```python
from build123d import *

# Parameters (mm, degrees)
BOSS_EXTRUDE1_DEPTH      = 2
BOSS_EXTRUDE1_DEPTH_BACK = 3
SKETCH1_W                = 120
SKETCH1_H                = 120
SKETCH3_W                = 27.75
SKETCH3_H                = 16.75
BOSS_EXTRUDE4_DEPTH      = 18
SKETCH4_W                = 23.75
SKETCH4_H                = 12.75
CUT_EXTRUDE1_DEPTH       = 18
SKETCH5_R                = 3
BOSS_EXTRUDE5_DEPTH      = 7
SKETCH6_W                = 10
SKETCH6_H                = 5
CUT_EXTRUDE2_DEPTH       = 2
SKETCH7_W                = 10
SKETCH7_H                = 5
CUT_EXTRUDE3_DEPTH       = 2
BOSS_EXTRUDE6_REACH      = 112.411
BOSS_EXTRUDE7_REACH      = 121.478
SKETCH12_W               = 120
SKETCH12_H               = 5
CUT_EXTRUDE4_DEPTH       = 3
SKETCH13_W               = 120
SKETCH13_H               = 5
CUT_EXTRUDE5_DEPTH       = 3
SKETCH14_W               = 114
SKETCH14_H               = 5
CUT_EXTRUDE6_DEPTH       = 3
SKETCH15_W               = 114
SKETCH15_H               = 5
CUT_EXTRUDE7_DEPTH       = 3
BOSS_EXTRUDE8_DEPTH      = 2


with BuildPart() as part:
    # Sketch1 → Boss-Extrude1 (new, two sides: drawn at the far end of the back side and taken through both)
    with BuildSketch(Plane(origin=(0, 0, 0), x_dir=(1, 0, 0), z_dir=(0, 1, 0)).offset(-BOSS_EXTRUDE1_DEPTH_BACK)):
        Rectangle(SKETCH1_W, SKETCH1_H)
    extrude(amount=BOSS_EXTRUDE1_DEPTH + BOSS_EXTRUDE1_DEPTH_BACK)

    # Sketch3 → Boss-Extrude4 (add)
    with BuildSketch(Plane(origin=(0, 0, 0), x_dir=(1, 0, 0), z_dir=(0, 1, 0))):
        with Locations((-43.125, -48.625)):
            Rectangle(SKETCH3_W, SKETCH3_H)
        with Locations((43.125, -48.625)):
            Rectangle(SKETCH3_W, SKETCH3_H)
        with Locations((43.125, 48.625)):
            Rectangle(SKETCH3_W, SKETCH3_H)
        with Locations((-43.125, 48.625)):
            Rectangle(SKETCH3_W, SKETCH3_H)
    extrude(amount=-BOSS_EXTRUDE4_DEPTH)

    # Sketch4 → Cut-Extrude1 (cut)
    with BuildSketch(Plane(origin=(0, 2, 0), x_dir=(1, 0, 0), z_dir=(0, 1, 0))):
        with Locations((-43.125, -48.625)):
            Rectangle(SKETCH4_W, SKETCH4_H)
        with Locations((43.125, -48.625)):
            Rectangle(SKETCH4_W, SKETCH4_H)
        with Locations((43.125, 48.625)):
            Rectangle(SKETCH4_W, SKETCH4_H)
        with Locations((-43.125, 48.625)):
            Rectangle(SKETCH4_W, SKETCH4_H)
    extrude(amount=-CUT_EXTRUDE1_DEPTH, mode=Mode.SUBTRACT)

    # Sketch5 → Boss-Extrude5 (add)
    with BuildSketch(Plane(origin=(0, -18, 0), x_dir=(-1, 0, 0), z_dir=(0, -1, 0))):
        with Locations(Location((48.5, -48.625, 0), (0, 0, 90))):
            Circle(SKETCH5_R)
        with Locations(Location((-48.5, -48.625, 0), (0, 0, 270))):
            Circle(SKETCH5_R)
        with Locations(Location((48.5, 48.625, 0), (0, 0, 270))):
            Circle(SKETCH5_R)
        with Locations(Location((-48.5, 48.625, 0), (0, 0, 270))):
            Circle(SKETCH5_R)
    extrude(amount=BOSS_EXTRUDE5_DEPTH)

    # Sketch6 → Cut-Extrude2 (cut)
    with BuildSketch(Plane(origin=(57, 0, 0), x_dir=(0, 0, -1), z_dir=(1, 0, 0))):
        with Locations((-48.625, -13.5)):
            Rectangle(SKETCH6_W, SKETCH6_H)
        with Locations((48.625, -13.5)):
            Rectangle(SKETCH6_W, SKETCH6_H)
    extrude(amount=-CUT_EXTRUDE2_DEPTH, mode=Mode.SUBTRACT)

    # Sketch7 → Cut-Extrude3 (cut)
    with BuildSketch(Plane.ZY.offset(57)):
        with Locations((48.625, -13.5)):
            Rectangle(SKETCH7_W, SKETCH7_H)
        with Locations((-48.625, -13.5)):
            Rectangle(SKETCH7_W, SKETCH7_H)
    extrude(amount=-CUT_EXTRUDE3_DEPTH, mode=Mode.SUBTRACT)

    # Sketch9 → Boss-Extrude6 (add, up to next)
    with BuildSketch(Plane(origin=(-29.25, 0, 0), x_dir=(0, 0, -1), z_dir=(1, 0, 0)), mode=Mode.PRIVATE) as boss_extrude6_sk1:
        Polygon((57, -3), (55, -3), (56.5, -18), (57, -18), align=None)
    boss_extrude6_tool1 = extrude(boss_extrude6_sk1.sketch, amount=BOSS_EXTRUDE6_REACH, mode=Mode.PRIVATE) - part.part
    # Sketch9 → Boss-Extrude6 (add, up to next)
    with BuildSketch(Plane(origin=(-29.25, 0, 0), x_dir=(0, 0, -1), z_dir=(1, 0, 0)), mode=Mode.PRIVATE) as boss_extrude6_sk2:
        Polygon((-56.5, -18), (-55, -3), (-57, -3), (-57, -18), align=None)
    boss_extrude6_tool2 = extrude(boss_extrude6_sk2.sketch, amount=BOSS_EXTRUDE6_REACH, mode=Mode.PRIVATE) - part.part
    add(boss_extrude6_tool1.solids().sort_by_distance((-29.25, -9, -56.3))[0])
    add(boss_extrude6_tool2.solids().sort_by_distance((-29.25, -9, 56.3))[0])

    # Sketch10 → Boss-Extrude7 (add, up to next)
    with BuildSketch(Plane.XY.offset(-40.25), mode=Mode.PRIVATE) as boss_extrude7_sk1:
        Polygon((-57, -3), (-54, -3), (-56.5, -18), (-57, -18), align=None)
    boss_extrude7_tool1 = extrude(boss_extrude7_sk1.sketch, amount=BOSS_EXTRUDE7_REACH, mode=Mode.PRIVATE) - part.part
    # Sketch10 → Boss-Extrude7 (add, up to next)
    with BuildSketch(Plane.XY.offset(-40.25), mode=Mode.PRIVATE) as boss_extrude7_sk2:
        Polygon((54, -3), (56.5, -18), (57, -18), (57, -3), align=None)
    boss_extrude7_tool2 = extrude(boss_extrude7_sk2.sketch, amount=BOSS_EXTRUDE7_REACH, mode=Mode.PRIVATE) - part.part
    add(boss_extrude7_tool1.solids().sort_by_distance((-55.97619, -8.714286, -40.25))[0])
    add(boss_extrude7_tool2.solids().sort_by_distance((55.97619, -8.714286, -40.25))[0])

    # Sketch12 → Cut-Extrude4 (cut)
    with BuildSketch(Plane.XY.offset(60)):
        with Locations((0, -0.5)):
            Rectangle(SKETCH12_W, SKETCH12_H)
    extrude(amount=-CUT_EXTRUDE4_DEPTH, mode=Mode.SUBTRACT)

    # Sketch13 → Cut-Extrude5 (cut)
    with BuildSketch(Plane(origin=(0, 0, -60), x_dir=(-1, 0, 0), z_dir=(0, 0, -1))):
        with Locations((0, -0.5)):
            Rectangle(SKETCH13_W, SKETCH13_H)
    extrude(amount=-CUT_EXTRUDE5_DEPTH, mode=Mode.SUBTRACT)

    # Sketch14 → Cut-Extrude6 (cut)
    with BuildSketch(Plane.ZY.offset(60)):
        with Locations((0, -0.5)):
            Rectangle(SKETCH14_W, SKETCH14_H)
    extrude(amount=-CUT_EXTRUDE6_DEPTH, mode=Mode.SUBTRACT)

    # Sketch15 → Cut-Extrude7 (cut)
    with BuildSketch(Plane(origin=(60, 0, 0), x_dir=(0, 0, -1), z_dir=(1, 0, 0))):
        with Locations((0, -0.5)):
            Rectangle(SKETCH15_W, SKETCH15_H)
    extrude(amount=-CUT_EXTRUDE7_DEPTH, mode=Mode.SUBTRACT)

    # Sketch16 → Boss-Extrude8 (add)
    with BuildSketch(Plane(origin=(0, 0, 0), x_dir=(1, 0, 0), z_dir=(0, 1, 0))):
        Polygon((-57, 47), (-67, 47), (-67, 67), (-47, 67), (-47, 57), (-57, 57), align=None)
        Polygon((57, 47), (57, 57), (47, 57), (47, 67), (67, 67), (67, 47), align=None)
        Polygon((67, -67), (47, -67), (47, -57), (57, -57), (57, -47), (67, -47), align=None)
        Polygon((-57, -57), (-47, -57), (-47, -67), (-67, -67), (-67, -47), (-57, -47), align=None)
    extrude(amount=BOSS_EXTRUDE8_DEPTH)


solid = part.part
```
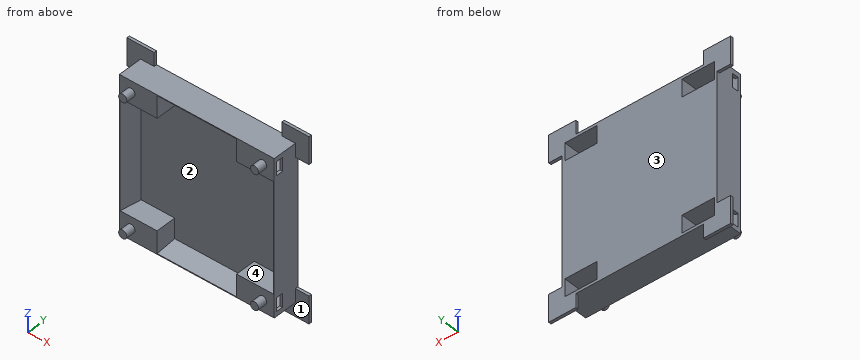
Can you work these out from the model? Positions are in its coordinate system, mm. Face numbers are marked on the shaded views. A direction names the side the tool comes from. Coordinates: 2 decimals unless noted, no trailing zeros. Loops run counter-clockwise (first coordinate to the right, second up) from the corner with the lowest first, then second, coordinate; pieces in that order, holes last. Notation, with made-up numbers: M -30.75,63 L -4.75,63 A34 cw -4.75,102 Z; hole C 48,-34.5 d7. An arc over 180 degrees is marked long. Put each result on its own line as item: value. Start each with the question number.
(1) Imagine slicing it at B-B on x = -9.5. List the corners of the cut face in (y, z) for me, and give its area (4 significant figures).
(2) I need wall thicknesses on probe 1 along Z at (x, y) = (35, -11.5); probe 2 along X at (y, z) = (-13.75, 54); probe 3 along X at (y, z) = (-5, 41.5). Which ranges of each line are inside material? Lowest first, please.
(3) Which directions (+Z, -Z, +X, -X, +Y, -Y) give clear straight access to the entire face, cutting with the end or side of a thin tool? Please do the marked faces 3 and 4.
(4) Imagine slicing it at A-A on z = 15. List the corners of the cut face in (x, y) for me, and give its area (4 significant figures).
(5) Imagine slicing it at C-C on y = -6.25. Give the number of separate pieces and of enclosed holes in the cut face, and give its area (3 significant figures).
(6) Will these pins go through, and if not, where does the flat tip stop? pin 1 Ø3 at (x, z) = (-10.5, -40.5) entering from -Y; pin 2 Ø7.5 at (x, y) = (38.5, -11) entering from -Z; pin 3 Ø10 at (x, z) = (53, -61.5) entering from -Y.
(7) We'd pull the mould along X, two halves only. Please class the marked faces 1 and 2: +X half, -X half, draft (parallel to the pull), parting line (faces both ways), or undercut.
(8) Imagine slicing it at D-D on y = -20. List the corners of the cut face in (x, z) for me (3 decimals), and give its area (3 significant figures).
Worked answers:
1. outline: M -18,-57 L 2,-57 L 2,57 L -18,57 L -18,56.5 L -3,55 L -3,-55 L -18,-56.5 Z
1. area: 607.5 mm2
2. probe 1: z = -57 to -55, -42.25 to -40.25, 40.25 to 42.25, 55 to 57
2. probe 2: x = -57 to -55, -31.25 to -29.25, 29.25 to 31.25, 55 to 57
2. probe 3: x = -57 to -29.25, 29.25 to 57
3. face 3: +Z, -Z, +X, -X, +Y
3. face 4: -Y
4. outline: M -57,-18 L -56.5,-18 L -54,-3 L 54,-3 L 56.5,-18 L 57,-18 L 57,2 L -57,2 Z
4. area: 622.5 mm2
5. separate pieces: 1
5. enclosed holes: 5
5. area: 1,240 mm2
6. pin 1: stops at y = -3
6. pin 2: stops at z = -57
6. pin 3: stops at y = -18
7. face 1: draft
7. face 2: undercut
8. outline: C -48.5,-48.625 d6; C -48.5,48.625 d6; C 48.5,-48.625 d6; C 48.5,48.625 d6
8. area: 113 mm2
